Geometry: final body of the model. Coordinates: model frame, mm. A direction names the side the tool comes from. Round coordinates to 2 decimals unless told otherwise and drop trailing zeros. Loops run counter-clockwise (first coordinate to the right, second up) from the corner with the lowest first, then second, coordinate; pieces in that order, holes last. Notation, with made-up numbers: (88.5, -9.5) -> (110.5, -9.5) arc R8 ccw to (110.5, 1.5) -> close; hole circle Ø8 at (48.5, 50). An arc over 180 degrees is marked (long way). Answer in a Markdown table with one row per item.
```python
from build123d import *

# Parameters (mm, degrees)
SKETCH1_R           = 2.4892
SKETCH1_R_2         = 2.667
SKETCH1_R_3         = 1.524
SKETCH1_R_4         = 11.522750336
BOSS_EXTRUDE1_DEPTH = 4.7625
SKETCH2_R           = 1.1303
CUT_EXTRUDE1_DEPTH  = 6.35


with BuildPart() as part:
    # Sketch1 → Boss-Extrude1 (new body)
    with BuildSketch(Plane(origin=(0, 0, 0), x_dir=(0, 0, -1), z_dir=(1, 0, 0))):
        with BuildLine():
            Line((-28.170295117, 0), (77.382795117, 0))
            ThreePointArc((77.382795117, 0), (79.627859148, 0.92993597), (80.557795117, 3.175))
            Line((80.557795117, 3.175), (80.557795117, 40.132))
            Line((80.557795117, 40.132), (84.771740045, 79.196103092))
            ThreePointArc((84.771740045, 79.196103092), (84.816236398, 80.272287311), (84.718413682, 81.344939685))
            Line((84.718413682, 81.344939685), (79.457064092, 114.563793628))
            Line((79.457064092, 114.563793628), (70.049332648, 113.073755348))
            Line((70.049332648, 113.073755348), (70.794351787, 108.369889626))
            Line((70.794351787, 108.369889626), (64.522530825, 107.376530773))
            Line((64.522530825, 107.376530773), (65.123512931, 103.582079091))
            Line((65.123512931, 103.582079091), (66.816904591, 103.850285981))
            Line((66.816904591, 103.850285981), (67.209281338, 101.372916701))
            Line((67.209281338, 101.372916701), (65.515889678, 101.10470981))
            Line((65.515889678, 101.10470981), (65.888399247, 98.752776949))
            Line((65.888399247, 98.752776949), (62.877925185, 98.2759647))
            Line((62.877925185, 98.2759647), (62.505415615, 100.627897561))
            Line((62.505415615, 100.627897561), (60.812023956, 100.359690671))
            Line((60.812023956, 100.359690671), (60.419647209, 102.837059951))
            Line((60.419647209, 102.837059951), (62.113038869, 103.105266841))
            Line((62.113038869, 103.105266841), (61.512056762, 106.899718524))
            Line((61.512056762, 106.899718524), (23.630258147, 100.899831052))
            Line((23.630258147, 100.899831052), (24.231240253, 97.105379369))
            Line((24.231240253, 97.105379369), (25.924631913, 97.373586259))
            Line((25.924631913, 97.373586259), (26.31700866, 94.896216979))
            Line((26.31700866, 94.896216979), (24.623617, 94.628010089))
            Line((24.623617, 94.628010089), (24.99612657, 92.276077228))
            Line((24.99612657, 92.276077228), (21.985652508, 91.799264978))
            Line((21.985652508, 91.799264978), (21.613142938, 94.151197839))
            Line((21.613142938, 94.151197839), (19.919751278, 93.882990949))
            Line((19.919751278, 93.882990949), (19.527374531, 96.360360229))
            Line((19.527374531, 96.360360229), (21.220766191, 96.62856712))
            Line((21.220766191, 96.62856712), (20.619784085, 100.423018802))
            Line((20.619784085, 100.423018802), (14.347963122, 99.429659949))
            Line((14.347963122, 99.429659949), (13.602943983, 104.133525671))
            Line((13.602943983, 104.133525671), (4.195212538, 102.643487392))
            ThreePointArc((4.195212538, 102.643487392), (2.66000635, 103.076460316), (1.992204883, 104.52503368))
            Line((1.992204883, 104.52503368), (1.992204883, 110.875))
            ThreePointArc((1.992204883, 110.875), (-0.797603027, 117.610192091), (-7.532795117, 120.4))
            Line((-7.532795117, 120.4), (-42.707795117, 120.4))
            ThreePointArc((-42.707795117, 120.4), (-69.471786785, 109.313991668), (-80.557795117, 82.55))
            Line((-80.557795117, 82.55), (-80.557795117, 50.292))
            Line((-80.557795117, 50.292), (-75.795295117, 50.292))
            Line((-75.795295117, 50.292), (-75.795295117, 40.132))
            Line((-75.795295117, 40.132), (-31.345295117, 40.132))
            Line((-31.345295117, 40.132), (-31.345295117, 3.175))
            ThreePointArc((-31.345295117, 3.175), (-30.415359148, 0.92993597), (-28.170295117, 0))
        make_face()
        with Locations(Location((-55.209041359, 60.43939525, 0), (0, 0, 180))):
            Circle(SKETCH1_R, mode=Mode.SUBTRACT)
        with Locations(Location((-14.692204883, 20.066, 0), (0, 0, 180))):
            Circle(SKETCH1_R_2, mode=Mode.SUBTRACT)
        with Locations(Location((-20.597190367, 70.048753759, 0), (0, 0, 180))):
            Circle(SKETCH1_R, mode=Mode.SUBTRACT)
        with Locations(Location((-64.818399868, 95.051246241, 0), (0, 0, 180))):
            Circle(SKETCH1_R, mode=Mode.SUBTRACT)
        with Locations(Location((-30.206548876, 104.66060475, 0), (0, 0, 180))):
            Circle(SKETCH1_R, mode=Mode.SUBTRACT)
        with Locations(Location((-78.176545117, 55.372, 0), (0, 0, 180))):
            Circle(SKETCH1_R_3, mode=Mode.SUBTRACT)
        with Locations(Location((-42.707795117, 82.55, 0), (0, 0, 180))):
            Circle(SKETCH1_R_4, mode=Mode.SUBTRACT)
        with Locations(Location((-7.532795117, 110.875, 0), (0, 0, 180))):
            Circle(SKETCH1_R, mode=Mode.SUBTRACT)
        with Locations(Location((76.243236649, 104.411043044, 0), (0, 0, 180))):
            Circle(SKETCH1_R_3, mode=Mode.SUBTRACT)
        with BuildLine():
            Line((65.317795117, 15.2273), (65.063795117, 15.2273))
            ThreePointArc((65.063795117, 15.2273), (60.225095117, 20.066), (65.063795117, 24.9047))
            Line((65.063795117, 24.9047), (65.317795117, 24.9047))
            ThreePointArc((65.317795117, 24.9047), (70.156495117, 20.066), (65.317795117, 15.2273))
        make_face(mode=Mode.SUBTRACT)
        with BuildLine():
            Line((71.035861406, 86.549018926), (72.027193342, 80.289995416))
            ThreePointArc((72.027193342, 80.289995416), (72.057683184, 79.9556661), (72.043814352, 79.620235963))
            Line((72.043814352, 79.620235963), (68.302723543, 44.939584088))
            ThreePointArc((68.302723543, 44.939584088), (66.751491112, 42.866217372), (64.187855338, 43.230831164))
            Line((64.187855338, 43.230831164), (22.026684653, 77.057314107))
            ThreePointArc((22.026684653, 77.057314107), (21.161269703, 79.690326664), (23.218859921, 81.547211328))
            Line((23.218859921, 81.547211328), (68.12978948, 88.66040377))
            ThreePointArc((68.12978948, 88.66040377), (70.020107562, 88.206578551), (71.035861406, 86.549018926))
        make_face(mode=Mode.SUBTRACT)
    extrude(amount=BOSS_EXTRUDE1_DEPTH)

    # Sketch2 → Cut-Extrude1 (cut)
    with BuildSketch(Plane.XY.offset(75.795295117)):
        with Locations((2.38125, 45.212)):
            Circle(SKETCH2_R)
    extrude(amount=-CUT_EXTRUDE1_DEPTH, mode=Mode.SUBTRACT)


solid = part.part
```
Item 1: Section query B-B, the plane z = 48.5. Output: boundary loops of the cut face in (x, y), and give its area (3 significant figures).
Ans:
| item | result |
|---|---|
| outline | (0, 40.13) -> (4.76, 40.13) -> (4.76, 72.59) -> (0, 72.59) -> close; (0, 92.51) -> (4.76, 92.51) -> (4.76, 119.95) -> (0, 119.95) -> close |
| area | 285 mm2 |
Item 2: Mould query, pull axis Z, two halves, no side actions, for faces 5 (the flat face through (2, 50.292, 78)), 6 (the cylindrical face through (2.35, 22.67, 14.11)), 7 (the flat face through (2, 67, 80.558)). Classes: released by +Z, released by -Z, zero draft, split by the parting line, or undercut.
Ans:
| item | result |
|---|---|
| face 5 | zero draft |
| face 6 | undercut |
| face 7 | released by +Z |
Item 3: Ray query, L1, parallel to Z at x = 1.6, y = 77.5; L2, parallel to Z at x = 1.45, y = 69; L3, parallel to Z at x = 1.25, y = 5. Return the intervals inside material, ascending.
Ans:
| item | result |
|---|---|
| L1 | -84.59 to -71.82, -21.6 to 32.35, 53.06 to 80.56 |
| L2 | -83.67 to -70.9, -32.07 to 18.34, 22.85 to 80.56 |
| L3 | -80.56 to 31.35 |
Item 4: Set-up query: faces 1 (the flat face through (2.348, 85.054, -45.36)), 2 (the flat face through (2.35, 113.83, -74.82)), 3 (the flat face through (2, 120.4, 25)), 4 (the flat face through (2, 21, -80.558)). Return all of +Z, -Z, +X, -X, +Y, -Y with unobstructed straight access to the full face (end or side cutting, diameter ignored); none if empty.
Ans:
| item | result |
|---|---|
| face 1 | +X, -X |
| face 2 | +X, -X, +Y |
| face 3 | +Z, -Z, +X, -X, +Y |
| face 4 | -Z, +X, -X, -Y |
Item 5: First-contact query: P1, Ø2.5, axis at x = 3.5, y = 23, coming from the +Z side; P2, Ø1.8, axis at x = 2.38, y = 45.21, coming from the +Z side; P3, Ø1.4, axis at x = 1, y = 26.5, coming from the -Z side. Flat tips, straight axial feed; report the tip coordinate or a pass-through.
Ans:
| item | result |
|---|---|
| P1 | z = 31.35 |
| P2 | z = 69.45 |
| P3 | z = -80.56 |
Item 6: Section query A-A, the plane z = -44. Output: boundary loops of the cut face in (x, y), and give its area (3 significant figures).
Ans:
| item | result |
|---|---|
| outline | (0, 0) -> (4.76, 0) -> (4.76, 59.43) -> (0, 59.43) -> close; (0, 84.84) -> (4.76, 84.84) -> (4.76, 104.13) -> (0, 104.13) -> close |
| area | 375 mm2 |
